Autodesk Inventor part; units mm, degrees
ref_plane "Work Plane1" through (-98.813, 0, 0) normal (1, 0, 0) x (0, 0, -1)
ref_plane "YZ Plane" through (0, 0, 0) normal (1, 0, 0) x (0, 1, 0)
ref_plane "XZ Plane" through (0, 0, 0) normal (0, 1, 0) x (-1, 0, 0)
sketch "Sketch1" plane through (0, 0, 0) normal (0, 1, 0) x (-1, 0, 0)
  line L0 (0, 0) -> (197.626, 0)
  line L1 (197.626, 0) -> (197.626, -77.381)
  line L2 (197.626, -77.381) -> (0, -77.381)
  line L3 (0, -77.381) -> (0, 0)
  dimension "d0" = 197.626
  dimension "d1" = 77.381
extrude "Extrusion1" add sketch "Sketch1" along normal blind 4.763
sketch "Sketch2" plane through (0, 4.763, 0) normal (0, 1, 0) x (1, 0, 0)
  line L0 (0, 41.072) -> (0, 36.309)
  line L1 (0, 36.309) -> (-60.123, 36.309)
  line L2 (-60.123, 36.309) -> (-60.123, 41.072)
  line L3 (-60.123, 41.072) -> (0, 41.072)
  line L4 (-197.626, 41.072) -> (-197.626, 36.309)
  line L5 (-197.626, 36.309) -> (-137.503, 36.309)
  line L6 (-137.503, 36.309) -> (-137.503, 41.072)
  line L7 (-137.503, 41.072) -> (-197.626, 41.072)
  dimension "d6" = 4.763
  dimension "d7" = 60.123
extrude "Extrusion2" cut sketch "Sketch2" against normal blind 22
sketch "Sketch3" plane through (0, 0, 0) normal (1, 0, 0) x (0, 0, -1)
  line L0 (36.309, 3.572) -> (3.806, 3.572)
  line L1 (3.806, 3.572) -> (3.806, 1.191)
  line L2 (3.806, 1.191) -> (36.309, 1.191)
  line L3 (36.309, 3.572) -> (36.309, 1.191)
  line L4 (41.072, 3.572) -> (73.575, 3.572)
  line L5 (73.575, 3.572) -> (73.575, 1.191)
  line L6 (73.575, 1.191) -> (41.072, 1.191)
  line L7 (41.072, 3.572) -> (41.072, 1.191)
  dimension "d12" = 32.503
extrude "Extrusion3" add sketch "Sketch3" along normal blind 4.763
ref_plane "Work Plane1" through (-98.813, 0, 0) normal (1, 0, 0) x (0, 0, -1)
mirror "Mirror1" about plane through (-98.813, 0, 0) normal (1, 0, 0) of "Extrusion3"
properties part number "Sustainable Chair_V4 - Lateral Support" material "Foam Board - V3"
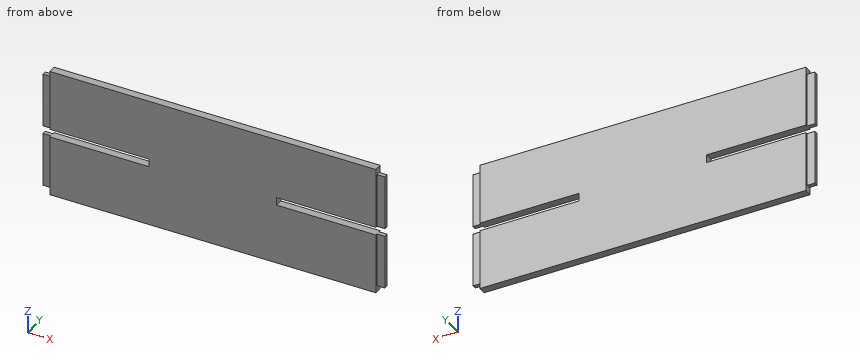
For this review, take the finished solid that the model builds, in its own axes (mm). Give positions to 0.01 mm unless a question says otherwise; leave off trailing zeros. Write each loop counter-clockwise with the first axis right and the second up, starting at its lowest first coordinate (ties: lowest second). Pieces come first, ordered by that corner, then holes.
Item 1: Take a section at C-C (y = 2.5). Give the boundary of the cut face in (x, z) (3 decimals).
Item 2: Insertion check: P1, Ø2.5, axis at x = -201, y = 2, coming from the -Z side (3 decimals); P2, Ø2.5, axis at y = 2, z = -39, coming from the -X side; P3, Ø5, axis at x = 3, z = -25.5, coming from the -Y side. Each pin has a flat end and moves straight along its axis. Give the tip position at first contact, or say it passes through.
Item 3: Take a section at A-A (x = -149.5). Give the boundary of the cut face in (y, z), and give its area (3 significant figures).
Item 4: Wall thickness on probe 1 along Z at (x, y) = (-15, 2.25); probe 2 along X at (y, z) = (4.3, -24.5): over which ranges is each line inside the solid? List them lowest first.
Item 5: Take a section at B-B (z = -28.5). Give the boundary of the cut face in (x, y), and give its area (3 significant figures).
Established:
1. outline: (-202.389, -73.575) - (-197.626, -73.575) - (-197.626, -77.381) - (0, -77.381) - (0, -73.575) - (4.763, -73.575) - (4.763, -41.072) - (-60.123, -41.072) - (-60.123, -36.309) - (4.763, -36.309) - (4.763, -3.806) - (0, -3.806) - (0, 0) - (-197.626, 0) - (-197.626, -3.806) - (-202.389, -3.806) - (-202.389, -36.309) - (-137.503, -36.309) - (-137.503, -41.072) - (-202.389, -41.072) - close
2. P1: stops at z = -73.575
2. P2: stops at x = -137.5
2. P3: stops at y = 1.19
3. outline: (0, -77.38) - (4.76, -77.38) - (4.76, -41.07) - (0, -41.07) - close; (0, -36.31) - (4.76, -36.31) - (4.76, 0) - (0, 0) - close
3. area: 346 mm2
4. probe 1: z = -77.38 to -41.07, -36.31 to 0
4. probe 2: x = -197.63 to 0
5. outline: (-202.39, 1.19) - (-197.63, 1.19) - (-197.63, 0) - (0, 0) - (0, 1.19) - (4.76, 1.19) - (4.76, 3.57) - (0, 3.57) - (0, 4.76) - (-197.63, 4.76) - (-197.63, 3.57) - (-202.39, 3.57) - close
5. area: 964 mm2
